```python
from build123d import *

# Parameters (mm, degrees)
F0_W     = 50.8
F0_H     = 127
F1_DEPTH = 6.35
F3_W     = 44.45
F3_H     = 12.7
F4_DEPTH = 50.8


with BuildPart() as f1:
    # F0 (on Front) → F1 (new body)
    with BuildSketch(Plane.XZ):
        Rectangle(F0_W, F0_H)
    extrude(amount=F1_DEPTH)

    # F3 (on face) → F4 (join)
    with BuildSketch(Plane.XZ.offset(6.35)):
        Rectangle(F3_W, F3_H)
    extrude(amount=F4_DEPTH)


solid = f1.part
```
Model file for the job. Use its own axes, mm. A direction names the side the tool comes from. Round coordinates to 2 decimals unless told otherwise and drop trailing zeros. Loops run counter-clockwise (first coordinate to the right, second up) from the corner with the lowest first, then second, coordinate; pieces in that order, holes last. Notation, with made-up numbers: M 73,36 L 102,36 A12 cw 102,59 Z; hole C -35.75,64.25 d9. An arc over 180 degrees is marked long. Put each result on its own line as item: value. Start each with the question number.
Item 1: Drop flat-ended pins along their axis: P1, Ø10, axis at y = -39.5, z = 1.5, coming from the -X side (3 decimals); P2, Ø6.5, axis at y = -28, z = -2.5, coming from the +X side (3 decimals); P3, Ø6, axis at x = -2, y = -41.5, coming from the +Z side. Give the stop position or say it passes through.
Item 2: Cut at A-A (x = 10.5). List the corners of the cut face in (y, z).
Item 3: 3-axis set-ups, long thin cutter, end or side, ignore diameter. For faces 4 (the face through (0, -57.15, 0)), 5 (the face through (-22.225, -31, 0)), 6 (the face through (22.225, -31, 0)): which of +Z, -Z, +X, -X, +Y, -Y reach the whole face in a straight line?
Item 4: Drill centre lines: line 1 along Z through (x, y) = (-1.5, -13); line 2 along X through (y, z) = (-24, -4) (3 decimals); line 3 along Y through (x, z) = (-22, -7). Where is each one in solid material? Low to high.
Item 5: Cut at B-B (y = -10). List the corners of the cut face in (x, z) (3 decimals), then the cut area to 3 significant figures.
Item 6: Cut at C-C (z = -42). List the corners of the cut face in (x, y).
Item 7: Mould opens along Z. For faces 1 (the face through (0, -31, -6.35)), 2 (the face through (0, -31, 6.35)), 3 (the face through (25.4, -3, -1)) say: released by +Z, released by -Z, zero draft, split by the parting line, or undercut.
Answer block:
1. P1: x = -22.225
1. P2: x = 22.225
1. P3: z = 6.35
2. outline: M -57.15,-6.35 L -6.35,-6.35 L -6.35,-63.5 L 0,-63.5 L 0,63.5 L -6.35,63.5 L -6.35,6.35 L -57.15,6.35 Z
3. face 4: +Z, -Z, +X, -X, -Y
3. face 5: +Z, -Z, -X, -Y
3. face 6: +Z, -Z, +X, -Y
4. line 1: -6.35 to 6.35
4. line 2: -22.225 to 22.225
4. line 3: -6.35 to 0
5. outline: M -22.225,-6.35 L 22.225,-6.35 L 22.225,6.35 L -22.225,6.35 Z
5. area: 565 mm2
6. outline: M -25.4,-6.35 L 25.4,-6.35 L 25.4,0 L -25.4,0 Z
7. face 1: released by -Z
7. face 2: released by +Z
7. face 3: zero draft
